Design review of the part built by this model. Coordinates are the model's own, in mm. Face numbers are marked on the shaded views. Give positions to 0.01 mm unless a question says otherwise; leave off trailing zeros. Write each loop counter-clockwise with the first axis right and the second up, starting at its lowest first coordinate (ties: lowest second). Pieces come first, ordered by that corner, then holes. Notation, with made-up numbers: M 85.25,-32.75 L 116.25,-32.75 A26 ccw 116.25,-7.75 Z; hole C 10.25,34 d1. An arc over 180 degrees is marked long. Answer in a Markdown table with one row per item.
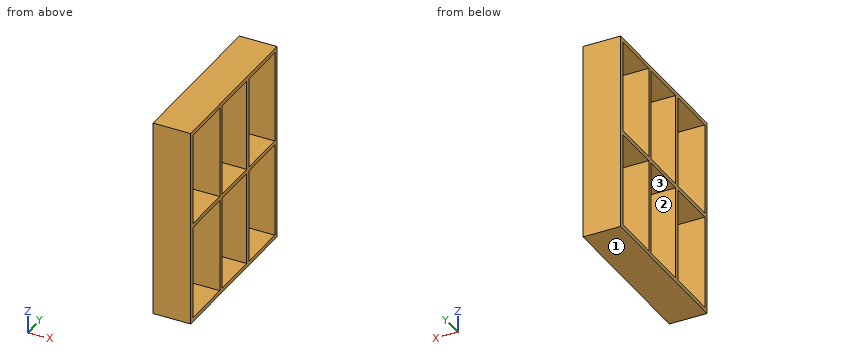
Autodesk Inventor part; units mm, degrees
ref_plane "YZ Plane" through (0, 0, 0) normal (1, 0, 0) x (0, 1, 0)
ref_plane "XZ Plane" through (0, 0, 0) normal (0, 1, 0) x (-1, 0, 0)
ref_plane "XY Plane" through (0, 0, 0) normal (0, 0, 1) x (1, 0, 0)
sketch "Sketch1" plane through (0, 0, 0) normal (1, 0, 0) x (0, 1, 0)
  line L0 (345.6873, 423.9836) -> (-90.3127, 423.9836)
  line L1 (-90.3127, 423.9836) -> (-90.3127, -104.0164)
  line L2 (-90.3127, -104.0164) -> (345.6873, -104.0164)
  line L3 (345.6873, -104.0164) -> (345.6873, 423.9836)
  line L4 (334.6873, -93.0164) -> (334.6873, 156.9836)
  line L5 (334.6873, 167.9836) -> (334.6873, 412.9836)
  line L6 (203.6873, 412.9836) -> (203.6873, 167.9836)
  line L7 (203.6873, 156.9836) -> (203.6873, -93.0164)
  line L8 (192.6873, 412.9836) -> (192.6873, 167.9836)
  line L9 (192.6873, 156.9836) -> (192.6873, -93.0164)
  line L10 (334.6873, 156.9836) -> (203.6873, 156.9836)
  line L11 (334.6873, 167.9836) -> (203.6873, 167.9836)
  line L12 (334.6873, 412.9836) -> (203.6873, 412.9836)
  line L13 (192.6873, 412.9836) -> (67.6873, 412.9836)
  line L14 (56.6873, 412.9836) -> (-79.3127, 412.9836)
  line L15 (192.6873, 156.9836) -> (67.6873, 156.9836)
  line L16 (56.6873, 156.9836) -> (-79.3127, 156.9836)
  line L17 (192.6873, 167.9836) -> (67.6873, 167.9836)
  line L18 (56.6873, 167.9836) -> (-79.3127, 167.9836)
  line L19 (56.6873, 412.9836) -> (56.6873, 167.9836)
  line L20 (56.6873, 156.9836) -> (56.6873, -93.0164)
  line L21 (67.6873, 412.9836) -> (67.6873, 167.9836)
  line L22 (67.6873, 156.9836) -> (67.6873, -93.0164)
  line L23 (-79.3127, -93.0164) -> (56.6873, -93.0164)
  line L24 (67.6873, -93.0164) -> (192.6873, -93.0164)
  line L25 (203.6873, -93.0164) -> (334.6873, -93.0164)
  line L26 (-79.3127, 412.9836) -> (-79.3127, 167.9836)
  line L27 (-79.3127, 156.9836) -> (-79.3127, -93.0164)
extrude "Extrusion1" add sketch "Sketch1" against normal blind 100
properties part number "Estanteria" material "Wood (Cherry)"
1) Add section B-B (x = -92). Write out the cut boundary in (y, z), and give its area (3 significant figures).
Geometry says:
| item | result |
|---|---|
| outline | M -90.31,-104.02 L 345.69,-104.02 L 345.69,423.98 L -90.31,423.98 Z; hole M -79.31,-93.02 L 56.69,-93.02 L 56.69,156.98 L -79.31,156.98 Z; hole M -79.31,167.98 L 56.69,167.98 L 56.69,412.98 L -79.31,412.98 Z; hole M 67.69,-93.02 L 192.69,-93.02 L 192.69,156.98 L 67.69,156.98 Z; hole M 67.69,167.98 L 192.69,167.98 L 192.69,412.98 L 67.69,412.98 Z; hole M 203.69,-93.02 L 334.69,-93.02 L 334.69,156.98 L 203.69,156.98 Z; hole M 203.69,167.98 L 334.69,167.98 L 334.69,412.98 L 203.69,412.98 Z |
| area | 36,200 mm^2 |
2) Add section C-C (z = 151). Write out the cut boundary in (x, y), and give its area (3 significant figures).
Geometry says:
| item | result |
|---|---|
| outline | M -100,-90.31 L 0,-90.31 L 0,-79.31 L -100,-79.31 Z; M -100,56.69 L 0,56.69 L 0,67.69 L -100,67.69 Z; M -100,192.69 L 0,192.69 L 0,203.69 L -100,203.69 Z; M -100,334.69 L 0,334.69 L 0,345.69 L -100,345.69 Z |
| area | 4,400 mm^2 |
3) Add section A-A (y = -44.5). Write out the cut boundary in (x, z).
Geometry says:
| item | result |
|---|---|
| outline | M -100,-104.02 L 0,-104.02 L 0,-93.02 L -100,-93.02 Z; M -100,156.98 L 0,156.98 L 0,167.98 L -100,167.98 Z; M -100,412.98 L 0,412.98 L 0,423.98 L -100,423.98 Z |
4) To check wall thickness, follow probe 1 along Z at (x, y) = (-62, 4); probe 2 along Y at (x, z) = (-68.5, -70). State the ranges of each line that lie inside material, in increasing order. Write a range as [from, to].
Geometry says:
| item | result |
|---|---|
| probe 1 | [-104.02, -93.02], [156.98, 167.98], [412.98, 423.98] |
| probe 2 | [-90.31, -79.31], [56.69, 67.69], [192.69, 203.69], [334.69, 345.69] |
5) The part is to be moulded in two halves that separate along Z. For the marked faces 1, 2 and 3, say which applies: released by +Z, released by -Z, zero draft, split by the parting line, or undercut.
Geometry says:
| item | result |
|---|---|
| face 1 | released by -Z |
| face 2 | undercut |
| face 3 | undercut |
